CAD build for the part. Positions are in the model's coordinates, mm. A direction names the side the tool comes from. Give positions to 0.01 mm unless a question says otherwise; leave off trailing zeros. Write each loop counter-clockwise with the first axis right and the second up, starting at its lowest first coordinate (ties: lowest second). Pieces come first, ordered by that corner, then holes. Notation, with made-up numbers: (-30.75, -2.75) - (17.25, -2.75) arc R7 ccw to (17.25, 4.25) - close; hole circle Ø3 at (52.25, -14). An arc over 180 degrees is marked (long way). Answer as a JSON object with one key per item and string values.
from build123d import *

# Parameters (mm, degrees)
CUT_EXTRUDE_7_DEPTH         = 185.932420089
CUT_EXTRUDE_7_DEPTH_BACK    = 185.932420089
SKETCH_10_W                 = 30
SKETCH_10_H                 = 10
SKETCH_14_R                 = 8
CUT_EXTRUDE_8_DEPTH         = 188.949461292
SKETCH_6_W                  = 18
SKETCH_6_H                  = 4
CUT_EXTRUDE_4_DEPTH         = 4
HOLE_WIZARD_20_0_20_1_D     = 20
HOLE_WIZARD_20_0_20_1_DEPTH = 35
HOLE_WIZARD_20_0_20_1_TIP   = 6.00860619
CHAMFER_3_SIZE              = 2
CHAMFER_4_SIZE              = 4


with BuildPart() as part:
    # Эскиз1 → Повернуть1 (revolve)
    with BuildSketch(Plane.XY, mode=Mode.PRIVATE) as revolve_1_sk:
        Polygon((0, 0), (0, 25), (80, 25), (80, 30), (120, 30), (120, 15), (180, 15), (180, 0), align=None)
    revolve(revolve_1_sk.sketch.rotate(Axis((0, 0, 0), (-1, 0, 0)), 90), axis=Axis((0, 0, 0), (-1, 0, 0)))

    # Эскиз10 → Вырез-Вытянуть7 (cut, two sides: drawn at the far end of the back side and taken through both)
    with BuildSketch(Plane.XY.offset(-CUT_EXTRUDE_7_DEPTH_BACK)):
        with Locations((55, 20)):
            Rectangle(SKETCH_10_W, SKETCH_10_H)
    extrude(amount=CUT_EXTRUDE_7_DEPTH + CUT_EXTRUDE_7_DEPTH_BACK, mode=Mode.SUBTRACT)

    # Эскиз14 → Вырез-Вытянуть8 (cut, through all)
    with BuildSketch(Plane(origin=(0, 15, 0), x_dir=(1, 0, 0), z_dir=(0, 1, 0))):
        with Locations(Location((55, 0, 0), (0, 0, 270))):
            Circle(SKETCH_14_R)
    extrude(amount=-CUT_EXTRUDE_8_DEPTH, mode=Mode.SUBTRACT)

    # Эскиз6 → Вырез-Вытянуть4 (cut, symmetric)
    with BuildSketch(Plane.XY):
        with Locations((146, 13)):
            Rectangle(SKETCH_6_W, SKETCH_6_H)
    extrude(amount=CUT_EXTRUDE_4_DEPTH, both=True, mode=Mode.SUBTRACT)

    # Диаметр отверстия Ø20.0 (20)1
    with Locations(Plane(origin=(0, 30, 0), x_dir=(1, 0, 0), z_dir=(0, 1, 0))):
        with Locations((100, 0)):
            Hole(HOLE_WIZARD_20_0_20_1_D / 2, depth=HOLE_WIZARD_20_0_20_1_DEPTH)
            with Locations((0, 0, -(HOLE_WIZARD_20_0_20_1_DEPTH + HOLE_WIZARD_20_0_20_1_TIP / 2))):  # 118° drill point
                Cone(0, HOLE_WIZARD_20_0_20_1_D / 2, HOLE_WIZARD_20_0_20_1_TIP, mode=Mode.SUBTRACT)

    # Фаска3
    chamfer_3_edges = [part.edges().sort_by_distance(p)[0] for p in [
        (180, 0, 15),
    ]]
    chamfer(chamfer_3_edges, length=CHAMFER_3_SIZE)

    # Фаска4
    chamfer_4_edges = [part.edges().sort_by_distance(p)[0] for p in [
        (0, 0, 25),
    ]]
    chamfer(chamfer_4_edges, length=CHAMFER_4_SIZE)


solid = part.part
(1) Flat gauge pins, fed straight in: P1, Ø12, axis at x = 123, y = -17, coming from the -Z side; P2, Ø3, axis at x = 145.5, y = 12, coming from the +Z side; P3, Ø15, axis at x = 51, z = 2.5, coming from the +Y side; P4, Ø5, axis at x = 56.5, z = 4.5, coming from the -Y side. Where does each tip first touch, or does it go through?
Answer key:
{"P1": "stops at z = -27.58", "P2": "stops at z = 10.71", "P3": "stops at y = 15", "P4": "passes through"}
(2) Probe L1, parallel to X at y = 18.5, z = 2.5; L2, parallel to Z at x = 100, y = 5; L3, parallel to Y at x = 133, z = 0.5. List the from-to ranges inside material, lowest first. Write a range as [from, to].
Answer key:
{"L1": "x = [0, 40], [70, 90.32], [109.68, 120]", "L2": "z = [-29.58, -10], [10, 29.58]", "L3": "y = [-14.99, 14.99]"}
(3) Saw through at A-A, the plane y = 0. Give the cut face in (x, z), and give its area (3 significant figures).
Answer key:
{"outline": "(0, -21) - (4, -25) - (80, -25) - (80, -30) - (120, -30) - (120, -15) - (178, -15) - (180, -13) - (180, 13) - (178, 15) - (120, 15) - (120, 30) - (80, 30) - (80, 25) - (4, 25) - (0, 21) - close; hole circle Ø16 at (55, 0); hole circle Ø20 at (100, 0)", "area": "7,660 mm²"}
(4) 3-axis set-ups, long thin cutter, end or side, ignore diameter. For faces 1 (the face through (100.28, -25.296, -16.128)), 2 (the face through (80, -25, -7)), 3 (the face through (48, 15, -5)), 4 (the face through (137, 13, 0)), 5 (the face through (120, -14, -6)): which of +Z, -Z, +X, -X, +Y, -Y reach the whole face in a straight line?
Answer key:
{"face 1": "+X, -X", "face 2": "-X", "face 3": "+Z, -Z, +Y", "face 4": "+Y", "face 5": "+X"}
(5) Saw through at D-D, the plane x = 17.5. Give the cut face in (y, z).
Answer key:
{"outline": "circle Ø50 at (0, 0)"}
(6) Pull direction X, two halves, no side cores. Call faces 6 (the face through (180, 0, 0)), 7 (the face through (146, 11, 0)), 8 (the face through (0.194, -6.366, -20.216)): pulls with the +X half, pulls with the -X half, needs draft (parallel to the pull), parting line crosses it, or undercut.
Answer key:
{"face 6": "pulls with the +X half", "face 7": "undercut", "face 8": "pulls with the -X half"}
(7) Saw through at B-B, the plane x = 55. Give the cut face in (y, z).
Answer key:
{"outline": "(-23.69, -8) arc R25 ccw to (15, -20) - (15, -8) - close; (-23.69, 8) - (15, 8) - (15, 20) arc R25 ccw to start"}
(8) Saw through at C-C, the plane x = 130. Give the cut face in (y, z).
Answer key:
{"outline": "circle Ø30 at (0, 0)"}
